Can you work these out from the drawing? Everything is in mm from the part's minimum corner. Coordinates: 2 decimals unless noted, no trailing zeros. Write each loop counter-clockwise with the first axis right and the second up, starting at its lowest first coordinate (ties: lowest second). Pieces come first, ordered by that corner, then holes. Notation, with made-up numbers: (-16, 80.5) -> (9, 80.5) arc R13 cw to (9, 85.5) -> close; hole circle Ø3 at (-22.75, 31.25). An arc over 180 degrees is marked (long way). Use a Markdown table: item, result. Add a question column.
Item 1: If I drill on line 1 along X through (y, z) = (2.05, 94.5); line 2 along X through (y, z) = (1.15, 170.5); line 3 along Z through (x, y) = (118.5, 1.55), over which ranges is the centre line in solid material (lowest first)? Write a range as from..to.
Item 2: Imagine slicing it at B-B, the plane z = 150. Write out the boundary of the cut face in (x, y), and give its area (3 significant figures).
Item 3: Imagine slicing it at C-C, the plane z = 129. Write out the boundary of the cut face in (x, y).
Item 4: Will this pin go through, and if not, where does the flat tip stop? pin 1 Ø6.5 at (x, z) = (55, 100) entering from -Y.
Item 5: Imagine slicing it at D-D, the plane y = 0.7. Count the separate pieces of the cut face and the enclosed holes in it, and give its area (3 significant figures).
Item 6: Imagine slicing it at A-A, the plane x = 190. Write out the boundary of the cut face in (y, z).
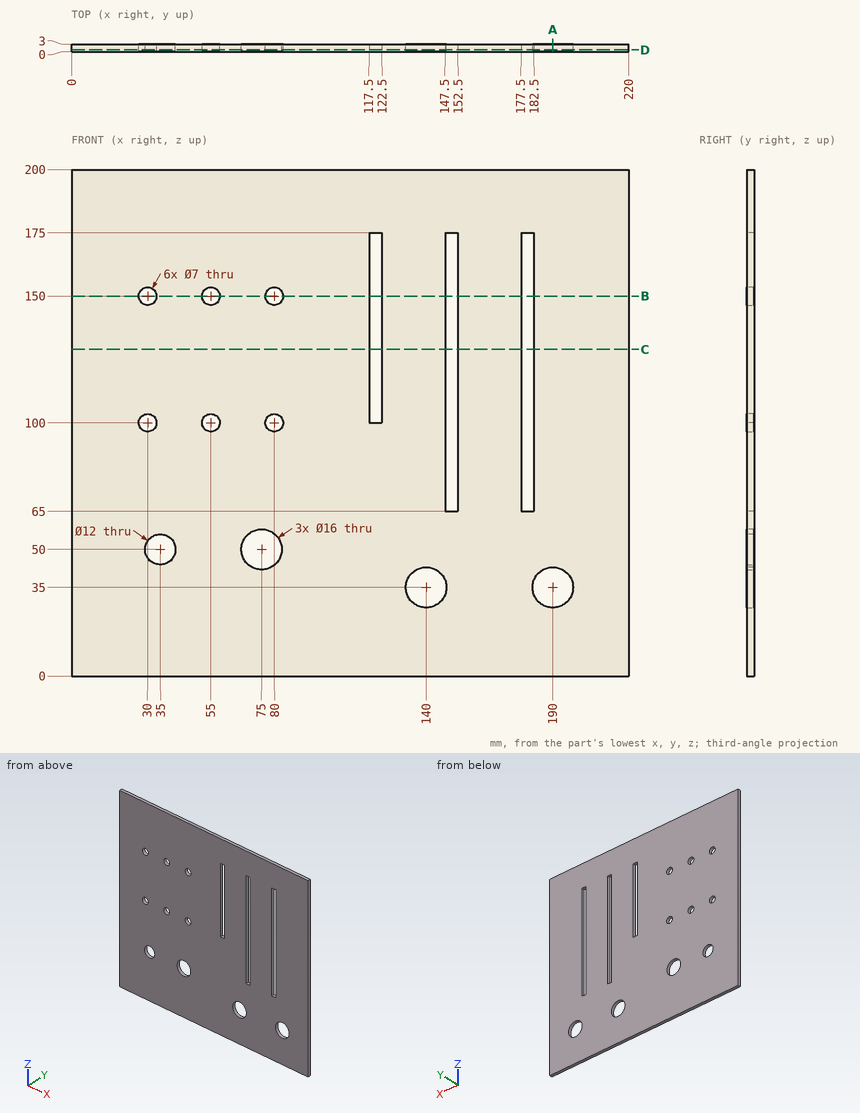
Ans:
| question | item | result |
|---|---|---|
| 1 | line 1 | x = 0..147.5, 152.5..177.5, 182.5..220 |
| 1 | line 2 | x = 0..117.5, 122.5..147.5, 152.5..177.5, 182.5..220 |
| 1 | line 3 | z = 0..100, 175..200 |
| 2 | outline | (0, 0) -> (26.5, 0) -> (26.5, 3) -> (0, 3) -> close; (33.5, 0) -> (51.5, 0) -> (51.5, 3) -> (33.5, 3) -> close; (58.5, 0) -> (76.5, 0) -> (76.5, 3) -> (58.5, 3) -> close; (83.5, 0) -> (117.5, 0) -> (117.5, 3) -> (83.5, 3) -> close; (122.5, 0) -> (147.5, 0) -> (147.5, 3) -> (122.5, 3) -> close; (152.5, 0) -> (177.5, 0) -> (177.5, 3) -> (152.5, 3) -> close; (182.5, 0) -> (220, 0) -> (220, 3) -> (182.5, 3) -> close |
| 2 | area | 552 mm^2 |
| 3 | outline | (0, 0) -> (117.5, 0) -> (117.5, 3) -> (0, 3) -> close; (122.5, 0) -> (147.5, 0) -> (147.5, 3) -> (122.5, 3) -> close; (152.5, 0) -> (177.5, 0) -> (177.5, 3) -> (152.5, 3) -> close; (182.5, 0) -> (220, 0) -> (220, 3) -> (182.5, 3) -> close |
| 4 | pin 1 | passes through |
| 5 | separate pieces | 1 |
| 5 | enclosed holes | 13 |
| 5 | area | 41,600 mm^2 |
| 6 | outline | (0, 0) -> (3, 0) -> (3, 27) -> (0, 27) -> close; (0, 43) -> (3, 43) -> (3, 200) -> (0, 200) -> close |
